from build123d import *

# Parameters (mm, degrees)
CUT_EXTRUDE1_DEPTH           = 33
CUT_EXTRUDE1_DEPTH_BACK      = 33
CUT_EXTRUDE2_DEPTH           = 33
CUT_EXTRUDE2_DEPTH_BACK      = 33
CUT_EXTRUDE3_DEPTH           = 33
CUT_EXTRUDE3_DEPTH_BACK      = 33
SKETCH5_W                    = 39.5
SKETCH5_H                    = 8
CUT_REVOLVE3_ANGLE           = 90
CUT_REVOLVE3_OTHER_WAY_ANGLE = 90


with BuildPart() as part:
    # Sketch1 → Revolve1 (revolve)
    with BuildSketch(Plane(origin=(0, 0, 0), x_dir=(0, 0, -1), z_dir=(1, 0, 0))):
        with BuildLine():
            Line((-19, 0), (-19, 32))
            Line((-19, 32), (35.444863729, 32))
            Line((35.444863729, 32), (40, 15))
            ThreePointArc((40, 15), (40.585786438, 13.585786438), (42, 13))
            Line((42, 13), (62.7, 13))
            ThreePointArc((62.7, 13), (63.619238816, 12.619238816), (64, 11.7))
            Line((64, 11.7), (64, 0))
            Line((64, 0), (-19, 0))
        make_face()
    revolve(axis=Axis((0, 0, -64), (0, 0, 1)))

    # Sketch2 → Cut-Extrude1 (cut, two sides)
    with BuildSketch(Plane(origin=(0, 0, 0), x_dir=(1, 0, 0), z_dir=(0, 1, 0))) as cut_extrude1_sk:
        Polygon((-8, 31), (-8, -20), (8, -20), (8, 31), (7, 32), (-7, 32), align=None)
    extrude(amount=CUT_EXTRUDE1_DEPTH, mode=Mode.SUBTRACT)
    extrude(cut_extrude1_sk.sketch, amount=-CUT_EXTRUDE1_DEPTH_BACK, mode=Mode.SUBTRACT)

    # Sketch3 → Cut-Extrude2 (cut, two sides)
    with BuildSketch(Plane(origin=(0, 0, 0), x_dir=(0, 0, -1), z_dir=(1, 0, 0))) as cut_extrude2_sk:
        Polygon((-52, -48), (64, -48), (64, -16), (-20, -16), (-20, 16), (64, 16), (64, 48), (-52, 48), align=None)
    extrude(amount=CUT_EXTRUDE2_DEPTH, mode=Mode.SUBTRACT)
    extrude(cut_extrude2_sk.sketch, amount=-CUT_EXTRUDE2_DEPTH_BACK, mode=Mode.SUBTRACT)

    # Sketch4 → Cut-Extrude3 (cut, two sides)
    with BuildSketch(Plane(origin=(0, 0, 0), x_dir=(1, 0, 0), z_dir=(0, 1, 0))) as cut_extrude3_sk:
        Polygon((-48, -52), (48, -52), (48, 64), (16, 64), (16, -20), (-16, -20), (-16, 64), (-48, 64), align=None)
    extrude(amount=CUT_EXTRUDE3_DEPTH, mode=Mode.SUBTRACT)
    extrude(cut_extrude3_sk.sketch, amount=-CUT_EXTRUDE3_DEPTH_BACK, mode=Mode.SUBTRACT)

    # Sketch5 → Cut-Revolve1 (revolve, cut)
    with BuildSketch(Plane.XY):
        with Locations((0, 4)):
            Rectangle(SKETCH5_W, SKETCH5_H)
    revolve(axis=Axis((19.75, 0, 0), (-1, 0, 0)), mode=Mode.SUBTRACT)

    # Sketch6 → Cut-Revolve2 (revolve, cut)
    with BuildSketch(Plane(origin=(0, 0, 0), x_dir=(0, 0, -1), z_dir=(1, 0, 0))):
        Polygon((30.9, 0), (30.9, 7.188), (63.288, 7.188), (64.1, 8), (64.1, 0), align=None)
    revolve(axis=Axis((0, 0, -64.1), (0, 0, 1)), mode=Mode.SUBTRACT)

    # Sketch7 → Cut-Revolve3 (revolve, cut)
    with BuildSketch(Plane(origin=(0, 0, 0), x_dir=(1, 0, 0), z_dir=(0, 1, 0))):
        Polygon((-19, -49.64182924), (0, -60.611484355), (19, -49.64182924), (19, -12.691412012), (0, -23.661067127), (-19, -12.691412012), align=None)
    revolve(axis=Axis((-19, 0, -32), (1, 0, 0)), revolution_arc=CUT_REVOLVE3_ANGLE, mode=Mode.SUBTRACT)

    # Sketch7 → Cut-Revolve3 other way (revolve, cut)
    with BuildSketch(Plane(origin=(0, 0, 0), x_dir=(1, 0, 0), z_dir=(0, 1, 0))):
        Polygon((-19, -49.64182924), (0, -60.611484355), (19, -49.64182924), (19, -12.691412012), (0, -23.661067127), (-19, -12.691412012), align=None)
    revolve(axis=Axis((-19, 0, -32), (-1, 0, 0)), revolution_arc=CUT_REVOLVE3_OTHER_WAY_ANGLE, mode=Mode.SUBTRACT)


solid = part.part
Here's how the part is built. I have some questions about the finished solid (model axes, mm). A direction names the side the tool comes from. Round coordinates to 2 decimals unless told otherwise and drop trailing zeros. Loops run counter-clockwise (first coordinate to the right, second up) from the corner with the lowest first, then second, coordinate; pieces in that order, holes last. Notation, with made-up numbers: M 5,13 L 29,13 A29 cw 29,33 Z; hole C 11,-4 d6. An arc over 180 degrees is marked long. Write each question's results on one line, items separated by ' | '. Start each with the question number.
(1) Thinking about a two-plate mould opening in X: for faces 4 (the conical face through (-12.056, 0.24, 16.7)), 5 (the flat face through (0, 10, -32)), 6 (the flat face through (2, 8, -64)), which applies, pulls with the +X half, pulls with the -X half, needs draft (parallel to the pull), parting line crosses it, or undercut?
(2) I want a section at A-A (x = 0). Please give me the cut outline in (y, z), then the cut area to 3 significant figures.
(3) I want a section at C-C (y = 0). State how many separate pieces and enclosed holes the cut face has, then the cut area to 3 significant figures.
(4) I want a section at D-D (z = -21). Please give me the cut outline in (x, y), then the cut area to 3 significant figures.
(5) I want a section at B-B (z = 0). Please give me the cut outline in (x, y).
(6) On a 3-axis mill with a long thin cutter (end or side, diameter ignored), from which of +Z, -Z, +X, -X, +Y, -Y can I reach the whole of each face in a straight line? I mean faces 1 (the flat face through (0, -11, -32)), 2 (the conical face through (11.944, 0.24, 16.765)), 3 (the cylindrical face through (7.91, -10.316, -52.495)). Say none if no direction works.
(7) Will these pins go through, and if not, where does the flat tip stop? P1, Ø8, axis at y = 9, z = -46.5, coming from the -X side; P2, Ø13, axis at y = 0, z = 0, coming from the -X side; P3, Ø5, axis at x = -6.5, z = -49.5, coming from the +Y side; P4, Ø12, axis at x = -0.5, y = -1.5, coming from the -Z side.
(8) If I drill on probe 1 along X at (y, z) = (-7.5, -26.5); probe 2 along Z at (x, y) = (5.5, 7.5); probe 3 along X at (y, z) = (-2, -41), over which ranges is the centre line in solid material (lowest first)? Write a range as from..to.
Solved:
1) face 4: pulls with the -X half | face 5: undercut | face 6: needs draft
2) outline: M -16,-39.73 L -15,-40 A2 cw -13,-42 L -13,-62.7 A1.3 ccw -11.7,-64 L -7.9,-64 L -7.19,-63.29 L -7.19,-32 L -16,-32 Z; M 7.19,-63.29 L 7.9,-64 L 11.7,-64 A1.3 ccw 13,-62.7 L 13,-42 A2 cw 15,-40 L 16,-39.73 L 16,-32 L 7.19,-32 Z | area: 420 mm²
3) separate pieces: 4 | enclosed holes: 0 | area: 945 mm²
4) outline: M -16,-16 L -8,-16 L -8,16 L -16,16 Z; M 8,-16 L 16,-16 L 16,16 L 8,16 Z | area: 512 mm²
5) outline: M -16,-16 L -8,-16 L -8,-8 L -16,-8 Z; M -16,8 L -8,8 L -8,16 L -16,16 Z; M 8,-16 L 16,-16 L 16,-8 L 8,-8 Z; M 8,8 L 16,8 L 16,16 L 8,16 Z
6) face 1: +Z, +Y, -Y | face 2: +Z, +X | face 3: -Z
7) P1: stops at x = -12 | P2: passes through | P3: stops at y = 12.37 | P4: stops at z = -63.68
8) probe 1: x = -16..-8, 8..16 | probe 2: z = -64..-32 | probe 3: x = -13.12..-6.9, 6.9..13.12
